Geometry: final body of the model. Coordinates: model frame, mm. Face numbers are marked on the shaded views. A direction names the side the tool comes from. Give positions to 0.01 mm unless a question says otherwise; leave off trailing zeros. Order: outer loops, then holes, each group sorted by start corner. A loop starts at its lowest first (then second) coordinate and runs counter-clockwise, first axis right, second up. Notation, with made-up numbers: (67.25, 88.25) - (112.25, 88.25) arc R10 cw to (112.25, 107.25) - close; hole circle Ø7 at (55.5, 80.5). An arc over 180 degrees is marked (long way). Use one line per item in the form item = value.
from build123d import *

# Parameters (mm, degrees)
F0_W     = 3.175
F0_H     = 6.6040001805
F0_H_2   = 3.81
F0_H_3   = 6.0959998195
F0_H_4   = 5.08
F1_DEPTH = 9.525
F0_R     = 3.3734375
F2_DEPTH = 9.525
F0_W_2   = 25.4
F3_DEPTH = 3.175
F4_START = -3.175
F4_DEPTH = 6.35
F5_R     = 2.032


# Not quite as in the source:
# - a feature names something its author has since deleted; it is built from what else it names


with BuildPart() as f1:
    # F0 (on Right) → F1 (new body)
    with BuildSketch(Plane.YZ):
        with Locations((23.2162721504, -5.0538677492)):
            Rectangle(F0_W, F0_H)
        with Locations((23.2162721504, -10.2608678395)):
            Rectangle(F0_W, F0_H_2)
        with Locations((23.2162721504, -19.1508678395)):
            Rectangle(F0_W, F0_H_2)
        with Locations((23.2162721504, -24.1038677492)):
            Rectangle(F0_W, F0_H_3)
        with Locations((23.2162721504, -14.7058678395)):
            Rectangle(F0_W, F0_H_4)
    extrude(amount=F1_DEPTH)



with BuildPart() as f1b:
    # F0 (on Right) → F1, piece 2 (new body)
    with BuildSketch(Plane.YZ):
        with Locations((-5.3587278496, -24.1038677492)):
            Rectangle(F0_W, F0_H_3)
        with Locations((-5.3587278496, -14.7058678395)):
            Rectangle(F0_W, F0_H_4)
        with Locations((-5.3587278496, -10.2608678395)):
            Rectangle(F0_W, F0_H_2)
        with Locations((-5.3587278496, -5.0538677492)):
            Rectangle(F0_W, F0_H)
        with Locations((-5.3587278496, -19.1508678395)):
            Rectangle(F0_W, F0_H_2)
    extrude(amount=F1_DEPTH)


with BuildPart() as f1_1:
    add(f1.part)

    add(f1b.part)  # F2 merges F1b
    # F0 (on Right) → F2 (join)
    with BuildSketch(Plane.YZ):
        Polygon((21.6287721504, -8.3558678395), (-3.7712278496, -8.3558678395), (-3.7712278496, -12.1658678395), (-3.7712278496, -17.2458678395), (-3.7712278496, -21.0558678395), (21.6287721504, -21.0558678395), (21.6287721504, -17.2458678395), (21.6287721504, -12.1658678395), align=None)
        with Locations((8.9287721504, -14.451867659)):
            Circle(F0_R, mode=Mode.SUBTRACT)
    extrude(amount=-F2_DEPTH)

    # F0 (on Right) → F3 (join)
    with BuildSketch(Plane.YZ):
        with Locations((8.9287721504, -5.0538677492)):
            Rectangle(F0_W_2, F0_H)
        Polygon((21.6287721504, -8.3558678395), (-3.7712278496, -8.3558678395), (-3.7712278496, -12.1658678395), (-3.7712278496, -17.2458678395), (-3.7712278496, -21.0558678395), (21.6287721504, -21.0558678395), (21.6287721504, -17.2458678395), (21.6287721504, -12.1658678395), align=None)
        with Locations((8.9287721504, -14.451867659)):
            Circle(F0_R, mode=Mode.SUBTRACT)
        with Locations((8.9287721504, -24.1038677492)):
            Rectangle(F0_W_2, F0_H_3)
    extrude(amount=F3_DEPTH)

    # F0 (on Right) → F4 (join)
    with BuildSketch(Plane.YZ.offset(F4_START)):
        with Locations((-5.3587278496, -14.7058678395)):
            Rectangle(F0_W, F0_H_4)
        with Locations((23.2162721504, -14.7058678395)):
            Rectangle(F0_W, F0_H_4)
        with Locations((23.2162721504, -19.1508678395)):
            Rectangle(F0_W, F0_H_2)
        with Locations((23.2162721504, -10.2608678395)):
            Rectangle(F0_W, F0_H_2)
        with Locations((-5.3587278496, -19.1508678395)):
            Rectangle(F0_W, F0_H_2)
        with Locations((-5.3587278496, -10.2608678395)):
            Rectangle(F0_W, F0_H_2)
    extrude(amount=-F4_DEPTH)

    # F5
    f5_edges = [f1_1.edges().sort_by_distance(p)[0] for p in [
        (-9.525, -6.946228, -14.705868),
        (-9.525, 24.803772, -14.705868),
    ]]
    fillet(f5_edges, radius=F5_R)


solid = f1_1.part
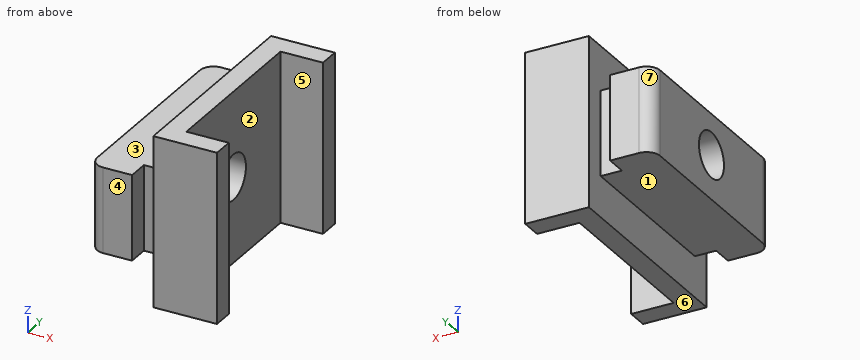
(1) Pull-direction query (Y, two-part tool) for the marked faces 4, 5, 6 and 7; classes: released by +Y, released by -Y, zero draft, split by the parting line, or undercut.
Computed values:
face_4 = released by -Y
face_5 = undercut
face_6 = zero draft
face_7 = released by +Y
(2) Contact query for flat-ended pins moving along their axis: pin 1 Ø5 at (x, y) = (-7, 4) entering from -Z; pin 2 Ø1 at (y, z) = (13, -12.5) entering from +X (3 decimals); pin 3 Ø3 at (x, y) = (6.5, 1.5) entering from -Z. Output: stop coordinate, or through.
Computed values:
pin_1 = -21.06
pin_2 = 3.175
pin_3 = through
(3) Cut plane B-B on z = -13.25. Output: boundary loops of the cut face in (x, y) (3 decimals), plus the area to 3 significant figures.
Computed values:
outline = (-9.525, -4.914) arc R2.032 ccw to (-7.493, -6.946) - (-3.175, -6.946) - (-3.175, -3.771) - (0, -3.771) - (0, -6.946) - (9.525, -6.946) - (9.525, -3.771) - (3.175, -3.771) - (3.175, 5.777) - (-9.525, 5.777) - close; (-9.525, 12.081) - (3.175, 12.081) - (3.175, 21.629) - (9.525, 21.629) - (9.525, 24.804) - (0, 24.804) - (0, 21.629) - (-3.175, 21.629) - (-3.175, 24.804) - (-7.493, 24.804) arc R2.032 ccw to (-9.525, 22.772) - close
area = 342 mm²
(4) Cut plane D-D on x = -1. Output: boundary loops of the cut face in (y, z).
Computed values:
outline = (-3.77, -21.06) - (21.63, -21.06) - (21.63, -8.36) - (-3.77, -8.36) - close; hole circle Ø6.75 at (8.93, -14.45)
(5) Reachability of the marked faces 1, 2 and 3 from +Z, -Z, +X, -X, +Y, -Y: full face, straight path, thin tool, end or side. Return the list, or none.
Computed values:
face_1 = -Z, -X, +Y, -Y
face_2 = +Z, -Z, +X
face_3 = +Z, -X, +Y, -Y
(6) Cut plane A-A on y = 19. Output: boundary loops of the cut face in (x, z) (3 decimals).
Computed values:
outline = (-9.525, -21.056) - (0, -21.056) - (0, -27.152) - (3.175, -27.152) - (3.175, -1.752) - (0, -1.752) - (0, -8.356) - (-9.525, -8.356) - close
(7) Ray query, line 1 along Y through (x, z) = (8.25, -17.25); line 2 along X through (y, z) = (-1, -8.75) (3 decimals); line 3 along Z through (x, y) = (-1.5, -2.5). Return the intervals inside material, ascending.
Computed values:
line_1 = -6.95 to -3.77, 21.63 to 24.8
line_2 = -9.525 to 3.175
line_3 = -21.06 to -8.36
(8) Cut plane C-C on z = -6.75. Output: boundary loops of the cut face in (x, y) (3 decimals), plus the area to 3 significant figures.
Computed values:
outline = (0, -6.946) - (9.525, -6.946) - (9.525, -3.771) - (3.175, -3.771) - (3.175, 21.629) - (9.525, 21.629) - (9.525, 24.804) - (0, 24.804) - close
area = 141 mm²
